from build123d import *

# Parameters (mm, degrees)
SKETCH1_R           = 25.825
SKETCH1_R_2         = 17.825
BOSS_EXTRUDE1_DEPTH = 40
SKETCH2_R           = 37.825
BOSS_EXTRUDE2_DEPTH = 8
SKETCH4_R           = 1.7
CUT_EXTRUDE2_DEPTH  = 9
SKETCH5_R           = 2.85
CUT_EXTRUDE3_DEPTH  = 4
FILLET1_R           = 2
SKETCH6_R           = 2.5
CUT_EXTRUDE4_DEPTH  = 9


with BuildPart() as part:
    # Sketch1 → Boss-Extrude1 (new body)
    with BuildSketch(Plane(origin=(0, 0, 0), x_dir=(1, 0, 0), z_dir=(0, 1, 0))):
        Circle(SKETCH1_R)
        Circle(SKETCH1_R_2, mode=Mode.SUBTRACT)
    extrude(amount=BOSS_EXTRUDE1_DEPTH)

    # Sketch2 → Boss-Extrude2 (add)
    with BuildSketch(Plane(origin=(0, 40, 0), x_dir=(1, 0, 0), z_dir=(0, 1, 0))):
        Circle(SKETCH2_R)
    extrude(amount=BOSS_EXTRUDE2_DEPTH)

    # Sketch4 → Cut-Extrude2 (cut, through all)
    with BuildSketch(Plane.XZ.offset(-40)):
        with Locations((0, 29.825)):
            Circle(SKETCH4_R)
        with Locations((29.825, 0)):
            Circle(SKETCH4_R)
        with Locations((0, -29.825)):
            Circle(SKETCH4_R)
        with Locations((-29.825, 0)):
            Circle(SKETCH4_R)
    extrude(amount=-CUT_EXTRUDE2_DEPTH, mode=Mode.SUBTRACT)

    # Sketch5 → Cut-Extrude3 (cut)
    with BuildSketch(Plane.XZ.offset(-40)):
        with Locations((0, 29.825)):
            Circle(SKETCH5_R)
        with Locations((29.825, 0)):
            Circle(SKETCH5_R)
        with Locations((0, -29.825)):
            Circle(SKETCH5_R)
        with Locations((-29.825, 0)):
            Circle(SKETCH5_R)
    extrude(amount=-CUT_EXTRUDE3_DEPTH, mode=Mode.SUBTRACT)

    # Fillet1
    fillet1_edges = [part.edges().sort_by_distance(p)[0] for p in [
        (-17.825, 0, 0),
    ]]
    fillet(fillet1_edges, radius=FILLET1_R)

    # Sketch6 → Cut-Extrude4 (cut, through all)
    with BuildSketch(Plane.XZ.offset(-40)):
        Circle(SKETCH6_R)
    extrude(amount=-CUT_EXTRUDE4_DEPTH, mode=Mode.SUBTRACT)


solid = part.part
Check sheet for the modelled part. Datum: model origin and axes. Units: mm. A direction names the side the tool comes from. Round coordinates to 2 decimals unless told otherwise and drop trailing zeros. Loops run counter-clockwise (first coordinate to the right, second up) from the corner with the lowest first, then second, coordinate; pieces in that order, holes last. Notation, with made-up numbers: M -22,-16 L 14,-16 A9 cw 14,1 Z; hole C 12.5,55.25 d9. An arc over 180 degrees is marked long. One line per item, written item: value.
(1) Sectioned sample at A-A, the plane x = 0. Count the separate pieces of the cut face and the enclosed holes in it, then the cut area to 3 significant figures.
Computed values:
separate pieces: 4
enclosed holes: 0
area: 1,130 mm^2
(2) Depth check by flat-ended pin: pin 1 Ø6.5 at (x, z) = (0.5, -30.5) entering from -Y; pin 2 Ø3.5 at (x, z) = (29.825, 0) entering from +Y; pin 3 Ø4 at (y, z) = (23, -8.5) entering from -X; pin 4 Ø2 at (x, y) = (-21, 33) entering from +Z. Enter the tip coordinate at first touch or a pass-through.
Computed values:
pin 1: stops at y = 40
pin 2: stops at y = 48
pin 3: stops at x = -24.99
pin 4: stops at z = 16.34
(3) Sectioned sample at D-D, the plane y = 6.5. Record the cut outline in (x, z) (3 decimals), then the cut area to 3 significant figures.
Computed values:
outline: C 0,0 d51.65; hole C 0,0 d35.65
area: 1,100 mm^2
(4) Access from +Z, -Z, +X, -X, +Y, -Y to the whole of each face (thin tool, end or side, straight path). Record for faces 1 (the face through (32, 44, 0)), 2 (the face through (8, 48, -1)).
Computed values:
face 1: -Y
face 2: +Z, -Z, +X, -X, +Y
(5) Sectioned sample at C-C, the plane z = 23. Record the cut outline in (x, y), then the cut area to 3 significant figures.
Computed values:
outline: M -30.03,40 L -11.74,40 L -11.74,0 L 11.74,0 L 11.74,40 L 30.03,40 L 30.03,48 L -30.03,48 Z
area: 1,420 mm^2
(6) Thickness scan on line 1 (Z direction, x = 0, y = 40.95) (3 decimals); line 2 (Z direction, x = 0, y = 31.5) (3 decimals); line 3 (Y direction, x = 9.5, z = 29). Record the ranges inside material, lowest first.
Computed values:
line 1: z = -37.825 to -32.675, -26.975 to -2.5, 2.5 to 26.975, 32.675 to 37.825
line 2: z = -25.825 to -17.825, 17.825 to 25.825
line 3: y = 40 to 48
(7) Release check for a two-part mould opening along Z. For faces 3 (the face through (36.08, 43.94, -11.36)), 4 (the face through (-0.04, 44, 27.96)), 5 (the face through (8, 0, 19)) record: +Z half, -Z half, draft (parallel to the pull), parting line (faces both ways), or undercut.
Computed values:
face 3: parting line
face 4: undercut
face 5: draft
